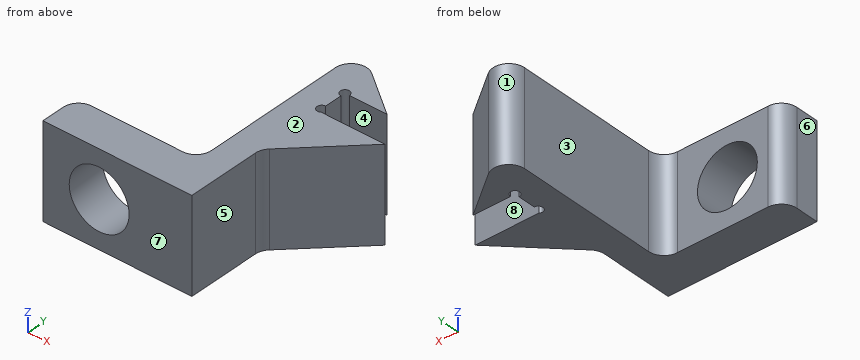
from build123d import *

# Parameters (mm, degrees)
BOSS_EXTRUDE1_DEPTH = 2.5
SKETCH4_R           = 1.6
CUT_EXTRUDE1_DEPTH  = 13.486214373


with BuildPart() as part:
    # Sketch3 → Boss-Extrude1 (new, symmetric)
    with BuildSketch(Plane.XY):
        with BuildLine():
            Line((-1.45304318, 2.879645015), (-1.45304318, 10.509737409))
            ThreePointArc((-1.45304318, 10.509737409), (-0.984259086, 11.268173328), (-0.096253627, 11.18798683))
            Line((-0.096253627, 11.18798683), (2.246891916, 9.43))
            Line((2.246891916, 9.43), (0.246891916, 9.43))
            ThreePointArc((0.246891916, 9.43), (-0.172404049, 9.603678075), (0.001274026, 9.18438211))
            Line((0.001274026, 9.18438211), (0.001274026, 8.242847777))
            ThreePointArc((0.001274026, 8.242847777), (-0.231933324, 7.920142408), (0.147658859, 7.8))
            Line((0.147658859, 7.8), (3.54695682, 7.8))
            Line((3.54695682, 7.8), (0.23979919, 4.492842832))
            ThreePointArc((0.23979919, 4.492842832), (0.062321779, 4.227229147), (0, 3.913916433))
            Line((0, 3.913916433), (0, 0))
            Line((0, 0), (-7.95, 0))
            Line((-7.95, 0), (-7.95, 1.239645015))
            ThreePointArc((-7.95, 1.239645015), (-7.709827561, 1.819472575), (-7.13, 2.059645015))
            Line((-7.13, 2.059645015), (-2.27304318, 2.059645015))
            ThreePointArc((-2.27304318, 2.059645015), (-1.69321562, 2.299817454), (-1.45304318, 2.879645015))
        make_face()
    extrude(amount=BOSS_EXTRUDE1_DEPTH, both=True)

    # Sketch4 → Cut-Extrude1 (cut, through all)
    with BuildSketch(Plane(origin=(0, 2.059645015, 0), x_dir=(1, 0, 0), z_dir=(0, 1, 0))):
        with Locations(Location((-4.95, 0, 0), (0, 0, 180))):
            Circle(SKETCH4_R)
    extrude(amount=-CUT_EXTRUDE1_DEPTH, mode=Mode.SUBTRACT)


solid = part.part
Model file for the job. Use its own axes, mm. Face numbers are marked on the shaded views. A direction names the side the tool comes from. Give positions to 0.01 mm unless a question says otherwise; leave off trailing zeros. Loops run counter-clockwise (first coordinate to the right, second up) from the corner with the lowest first, then second, coordinate; pieces in that order, holes last.
Item 1: Mould opens along Y. For the marked faces 6, 7 and 8 say: +Y half, -Y half, draft (parallel to the pull), parting line (faces both ways), or undercut.
Check values:
face 6: draft
face 7: -Y half
face 8: undercut
Item 2: Slice it at D-D (x = -2.5). Write the cut outline in (y, z).
Check values:
outline: (0, -2.5) - (2.06, -2.5) - (2.06, 2.5) - (0, 2.5) - close
Item 3: Slice it at B-B (x = -4.95). Write the cut outline in (y, z), plus the area to 3 significant figures.
Check values:
outline: (0, -2.5) - (2.06, -2.5) - (2.06, -1.6) - (0, -1.6) - close; (0, 1.6) - (2.06, 1.6) - (2.06, 2.5) - (0, 2.5) - close
area: 3.71 mm2
Item 4: Slice it at A-A (z = -1.95). Write the cut outline in (x, y).
Check values:
outline: (-7.95, 0) - (0, 0) - (0, 3.91) arc R0.82 cw to (0.24, 4.49) - (3.55, 7.8) - (0.15, 7.8) arc R0.25 cw (long way) to (0, 8.24) - (0, 9.18) arc R0.25 cw (long way) to (0.25, 9.43) - (2.25, 9.43) - (-0.1, 11.19) arc R0.85 ccw to (-1.45, 10.51) - (-1.45, 2.88) arc R0.82 cw to (-2.27, 2.06) - (-7.13, 2.06) arc R0.82 ccw to (-7.95, 1.24) - close
Item 5: Which spindle directions (+Z, -Z, +X, -X, +Y, -Y) get a long thin tool onto all of the face, cutting with end or side? Do the marked faces 1, 2, 3, 4 and 5. Say none if no direction does.
Check values:
face 1: +Z, -Z, +Y
face 2: +Z, +X, -X, +Y, -Y
face 3: +Z, -Z, -X, +Y
face 4: +Z, -Z, +X
face 5: +Z, -Z, +X, -Y
Item 6: Drill centre lines: line 1 along Z through (x, y) = (-4.95, 1.4); line 2 along Y through (x, z) = (0.75, -0.95); line 3 along X through (y, z) = (1.25, 1.3). Where is each one in solid material? Low to high.
Check values:
line 1: z = -2.5 to -1.6, 1.6 to 2.5
line 2: y = 5 to 7.8, 9.43 to 10.55
line 3: x = -7.95 to -5.88, -4.02 to 0
Item 7: Slice it at C-C (z = 0.25). Write the cut outline in (x, y), plus the area to 3 significant figures.
Check values:
outline: (-7.95, 0) - (-6.53, 0) - (-6.53, 2.06) - (-7.13, 2.06) arc R0.82 ccw to (-7.95, 1.24) - close; (-3.37, 0) - (0, 0) - (0, 3.91) arc R0.82 cw to (0.24, 4.49) - (3.55, 7.8) - (0.15, 7.8) arc R0.25 cw (long way) to (0, 8.24) - (0, 9.18) arc R0.25 cw (long way) to (0.25, 9.43) - (2.25, 9.43) - (-0.1, 11.19) arc R0.85 ccw to (-1.45, 10.51) - (-1.45, 2.88) arc R0.82 cw to (-2.27, 2.06) - (-3.37, 2.06) - close
area: 31.1 mm2
Item 8: Drop flat-ended pins along their axis: P1, Ø1.5, axis at y = 8.5, z = -0.5, coming from the -X side; P2, Ø1.6, axis at x = 1.5, z = 1, coming from the -Y side; P3, Ø2, axis at x = 2, z = 1.5, coming from the +Y side; P4, Ø5, axis at x = -6, y = 5.5, coming from the +Z side. Give the stop position or say it passes through.
Check values:
P1: stops at x = -1.45
P2: stops at y = 4.95
P3: stops at y = 10.37
P4: passes through
